CAD build for the part. Positions are in the model's coordinates, mm. Give positions to 0.01 mm unless a question says otherwise; leave off trailing zeros. Write each loop counter-clockwise with the first axis right and the second up, starting at its lowest first coordinate (ties: lowest second). Pieces come first, ordered by that corner, then holes. Notation, with made-up numbers: M -18.75,-20 L -8.75,-20 A19 ccw -8.75,-11 Z; hole C 60.25,-6.5 d10. An arc over 180 degrees is marked long. One line per question, with ' | ' between items. Start each with the question number.
1. Cut at B-B, the plane x = 3.5. Write the cut outline in (y, z), then the cut area to 3 significant figures.
2. Wall check: L1, parallel to Z at x = 10.75, y = -1.05; L2, parallel to Z at x = 7.5, y = -0.8; L3, parallel to X at y = -0.1, z = 0.5. Give the ranges that are in metal, low to high.
3. Pull direction X, two halves, no side cores. Call faces 1 (the face through (-1.307, -1, 4)), 2 (the face through (5, -1.27, -3)), 3 (the face through (6.444, -0.626, -5.498)): released by +X, released by -X, zero draft, split by the parting line, or undercut.
4. Cut at A-A, the plane z = -5.75. Write the cut outline in (x, y).
```python
from build123d import *

# Parameters (mm, degrees)
F1_DEPTH = 1.27


with BuildPart() as f1:
    # F0 (on Front) → F1 (new body)
    with BuildSketch(Plane.XZ):
        Polygon((11.8264406887, -10.7807891433), (-0.8713469764, 4.4592108567), (-1.5063469764, 4.4592108567), (-1.3065064559, 4.2193604502), (-1.0086600117, 3.8618824447), (-0.5849018199, 3.3532840169), (-0.2455411144, 2.9459802181), (0.0911234886, 2.541912306), (0.573246897, 1.9632634155), (0.928909441, 1.5363940023), (1.6323374241, 0.6921333527), (2.2090147436, 0), (2.8997819306, -0.8290650473), (3.321811547, -1.3355888232), (4.0407046407, -2.1984108389), (4.5513520585, -2.8112945043), (5.0631082221, -3.4255088966), (5.4507959484, -3.8908152243), (5.9248896017, -4.4598267298), (6.2394758554, -4.8373960067), (6.6537557336, -5.3346184765), (7.3379562236, -6.1558021144), (7.575495537, -6.4408989541), (8.2138098271, -7.2070095585), (8.5938442703, -7.6631303464), (9.035790701, -8.1935584635), (9.2577511046, -8.4599573544), (9.7840033839, -9.0915701163), (10.1199439716, -9.4947690587), (10.2986362516, -9.7092371549), (10.5988050888, -10.0695025176), (11.0456617549, -10.0695025176), (11.0605312511, -10.0695025176), (11.0605312511, -10.099911131), (11.0605312511, -10.1845458375), (11.0605312511, -10.2025323822), (11.0605312511, -10.7807891433), (11.1914406887, -10.7807891433), (11.2468553707, -10.7807891433), align=None)
        Polygon((-1.0086600117, 3.8618824447), (-1.3065064559, 4.2193604502), (-1.3065064559, 3.4027206711), align=None)
        Polygon((-0.5849018199, 3.3532840169), (-1.0086600117, 3.8618824447), (-0.7916077157, 2.1798356902), align=None)
        with BuildLine():
            Line((11.0456617549, -10.7807891433), (11.0605312511, -10.7807891433))
            Line((11.0605312511, -10.7807891433), (11.0605312511, -10.2025323822))
            Line((11.0605312511, -10.2025323822), (11.0605312511, -10.1845458375))
            Line((11.0605312511, -10.1845458375), (11.0605312511, -10.099911131))
            Line((11.0605312511, -10.099911131), (11.0456617549, -10.099911131))
            Line((11.0456617549, -10.099911131), (11.0456617549, -10.4917703344))
            ThreePointArc((11.0456617549, -10.4917703344), (11.0469379879, -10.5246867127), (11.0456617549, -10.557603091))
            Line((11.0456617549, -10.557603091), (11.0456617549, -10.7807891433))
        make_face()
        Polygon((-0.2455411144, 2.9459802181), (-0.5849018199, 3.3532840169), (-0.4268874764, 2.3943767883), align=None)
        Polygon((0.0911234886, 2.541912306), (-0.2455411144, 2.9459802181), (0, 2.0082029514), align=None)
        with BuildLine():
            Line((11.0456617549, -10.4917703344), (11.0456617549, -10.557603091))
            ThreePointArc((11.0456617549, -10.557603091), (11.0469379879, -10.5246867127), (11.0456617549, -10.4917703344))
        make_face()
        Polygon((0.573246897, 1.9632634155), (0.0911234886, 2.541912306), (0.277421379, 0.6077454309), (0.4825687985, 1.5477624331), align=None)
        with BuildLine():
            ThreePointArc((10.6390425935, -10.099911131), (10.9168146182, -10.2185735503), (11.0456617549, -10.4917703344))
            Line((11.0456617549, -10.4917703344), (11.0456617549, -10.099911131))
            Line((11.0456617549, -10.099911131), (10.6390425935, -10.099911131))
        make_face()
        Polygon((0.928909441, 1.5363940023), (0.573246897, 1.9632634155), (0.6398208604, 1.5715317733), (0.7435218431, 0.9613389266), align=None)
        Polygon((0.6398208604, 1.5715317733), (0.573246897, 1.9632634155), (0.4825687985, 1.5477624331), (0.5450948966, 1.1798490652), align=None)
        Polygon((10.6390425935, -10.099911131), (11.0456617549, -10.099911131), (11.0456617549, -10.0695025176), (10.5988050888, -10.0695025176), (10.6241411856, -10.099911131), align=None)
        Polygon((1.6323374241, 0.6921333527), (0.928909441, 1.5363940023), (1.3060569763, -0.1315863774), (1.4691972002, 0.2802734877), align=None)
        Polygon((10.3788425163, -10.099911131), (10.6241411856, -10.099911131), (10.5988050888, -10.0695025176), (10.3788425163, -10.0695025176), align=None)
        Polygon((2.2090147436, 0), (1.6323374241, 0.6921333527), (1.7359070743, 0.1199951858), (1.900736941, -0.7905559032), (2.0548758423, -0.3952779516), align=None)
        Polygon((1.7359070743, 0.1199951858), (1.6323374241, 0.6921333527), (1.4691972002, 0.2802734877), (1.6247893218, -0.2425153507), align=None)
        Polygon((10.3788425163, -10.0695025176), (10.5988050888, -10.0695025176), (10.2986362516, -9.7092371549), align=None)
        Polygon((2.8997819306, -0.8290650473), (2.2090147436, 0), (2.3425826603, -0.5337401752), (2.5757791009, -1.4655980049), align=None)
        Polygon((2.3425826603, -0.5337401752), (2.2090147436, 0), (2.0548758423, -0.3952779516), (2.2364195902, -0.8732591523), align=None)
        Polygon((10.1796239614, -9.9518895149), (10.2986362516, -9.7092371549), (10.1199439716, -9.4947690587), align=None)
        Polygon((3.321811547, -1.3355888232), (2.8997819306, -0.8290650473), (3.0238747131, -2.1357438527), align=None)
        Polygon((9.9704461172, -9.9947974086), (10.1199439716, -9.4947690587), (9.7840033839, -9.0915701163), (9.8473794647, -9.3926533487), (9.8465451714, -9.3945556409), align=None)
        Polygon((4.0407046407, -2.1984108389), (3.321811547, -1.3355888232), (3.7131523713, -3.757573897), (3.9366614966, -2.6936607331), align=None)
        Polygon((9.8465451714, -9.3945556409), (9.7840033839, -9.0915701163), (9.6553254332, -9.3716533956), (9.7383982677, -9.6411439871), align=None)
        Polygon((9.6553254332, -9.3716533956), (9.7840033839, -9.0915701163), (9.2577511046, -8.4599573544), (9.5855835825, -9.5234550536), align=None)
        Polygon((9.8473794647, -9.3926533487), (9.7840033839, -9.0915701163), (9.8465451714, -9.3945556409), align=None)
        Polygon((4.5513520585, -2.8112945043), (4.0407046407, -2.1984108389), (4.194536978, -2.7820212599), (4.3483693153, -3.3656316809), align=None)
        Polygon((4.194536978, -2.7820212599), (4.0407046407, -2.1984108389), (3.9366614966, -2.6936607331), (4.0082986512, -3.1370188198), align=None)
        Polygon((9.1757364571, -8.7760863826), (9.2577511046, -8.4599573544), (9.035790701, -8.1935584635), align=None)
        Polygon((5.0631082221, -3.4255088966), (4.5513520585, -2.8112945043), (4.8349178396, -4.1765468195), align=None)
        Polygon((8.8703604415, -9.041281417), (9.035790701, -8.1935584635), (8.5938442703, -7.6631303464), (8.6790014305, -8.0875519305), align=None)
        Polygon((5.4507959484, -3.8908152243), (5.0631082221, -3.4255088966), (5.3079519421, -4.3792752549), align=None)
        Polygon((8.6790014305, -8.0875519305), (8.5938442703, -7.6631303464), (8.4427986396, -7.9624497125), (8.5217449814, -8.4112593904), align=None)
        Polygon((8.4427986396, -7.9624497125), (8.5938442703, -7.6631303464), (8.2138098271, -7.2070095585), (8.291753009, -8.2617690787), align=None)
        Polygon((5.9248896017, -4.4598267298), (5.4507959484, -3.8908152243), (5.8080158196, -4.9604312517), align=None)
        Polygon((8.0737182871, -7.8651150689), (8.2138098271, -7.2070095585), (7.575495537, -6.4408989541), (7.7781930442, -7.0203286494), align=None)
        Polygon((6.2394758554, -4.8373960067), (5.9248896017, -4.4598267298), (6.1053512618, -5.2442513406), align=None)
        Polygon((7.7781930442, -7.0203286494), (7.575495537, -6.4408989541), (7.4394400226, -6.8352251344), (7.6648117974, -7.2927363217), align=None)
        Polygon((7.4394400226, -6.8352251344), (7.575495537, -6.4408989541), (7.3379562236, -6.1558021144), (7.3379562236, -7.1293530054), align=None)
        Polygon((6.6537557336, -5.3346184765), (6.2394758554, -4.8373960067), (6.6537557336, -6.1768037267), align=None)
        Polygon((7.1595408954, -6.6498368979), (7.3379562236, -6.1558021144), (6.6537557336, -5.3346184765), align=None)
    extrude(amount=F1_DEPTH)


solid = f1.part
```
Here are the results:
1) outline: M -1.27,-2.44 L 0,-2.44 L 0,-0.79 L -1.27,-0.79 Z | area: 2.10 mm^2
2) L1: -10.12 to -9.49 | L2: -6.96 to -5.59 | L3: 1.16 to 2.43
3) face 1: released by -X | face 2: zero draft | face 3: undercut
4) outline: M 6.52,-1.27 L 6.65,-1.27 L 6.65,0 L 6.52,0 Z; M 6.81,-1.27 L 7.63,-1.27 L 7.63,0 L 6.81,0 Z
